```python
from build123d import *

# Parameters (mm, degrees)
SKETCH2_W             = 10
SKETCH2_H             = 14
SKETCH2_R             = 2.1
BOSS_EXTRUDE1_DEPTH   = 5
BOSS_EXTRUDE1_2_DEPTH = 5
SKETCH3_W             = 44.5
SKETCH3_H             = 39
SKETCH3_W_2           = 14
SKETCH3_H_2           = 5
BOSS_EXTRUDE2_DEPTH   = 2
BOSS_EXTRUDE4_DEPTH   = 32
SKETCH5_W             = 2
SKETCH5_H             = 85
BOSS_EXTRUDE5_DEPTH   = 37
SKETCH6_W             = 14
SKETCH6_H             = 30
CUT_EXTRUDE1_DEPTH    = 200
SKETCH7_W             = 20
SKETCH7_H             = 20
CUT_EXTRUDE2_DEPTH    = 16
FILLET1_R             = 2
SKETCH8_W             = 119.619460544
SKETCH8_H             = 55.607641494
CUT_EXTRUDE3_DEPTH    = 32
SKETCH9_W             = 100
SKETCH9_H             = 35
BOSS_EXTRUDE6_DEPTH   = 2
SKETCH10_W            = 89
SKETCH10_H            = 4
CUT_EXTRUDE4_DEPTH    = 10
BOSS_EXTRUDE7_DEPTH   = 25
SKETCH12_W            = 2
SKETCH12_H            = 35
BOSS_EXTRUDE8_DEPTH   = 2
SKETCH13_W            = 104
SKETCH13_H            = 37
BOSS_EXTRUDE9_DEPTH   = 2
SKETCH14_W            = 13
SKETCH14_H            = 30
CUT_EXTRUDE5_DEPTH    = 104
SKETCH15_W            = 13
SKETCH15_H            = 25
CUT_EXTRUDE7_DEPTH    = 120


with BuildPart() as part:
    # Sketch2 → Boss-Extrude1 (new body)
    with BuildSketch(Plane(origin=(0, 0, 0), x_dir=(1, 0, 0), z_dir=(0, 1, 0))):
        with Locations((114.448385229, -132.360414745)):
            Rectangle(SKETCH2_W, SKETCH2_H)
        with Locations((114.448385229, -132.360414745)):
            Circle(SKETCH2_R, mode=Mode.SUBTRACT)
    extrude(amount=BOSS_EXTRUDE1_DEPTH)



with BuildPart() as body_2:
    # Sketch2 → Boss-Extrude1 2 (new body)
    with BuildSketch(Plane(origin=(0, 0, 0), x_dir=(1, 0, 0), z_dir=(0, 1, 0))):
        with Locations((114.448385229, -172.360414745)):
            Rectangle(SKETCH2_W, SKETCH2_H)
        with Locations((114.448385229, -172.360414745)):
            Circle(SKETCH2_R, mode=Mode.SUBTRACT)
    extrude(amount=BOSS_EXTRUDE1_2_DEPTH)


with BuildPart() as part_1:
    add(part.part)

    add(body_2.part)  # Boss-Extrude2 merges body 2
    # Sketch3 → Boss-Extrude2 (add)
    with BuildSketch(Plane(origin=(119.448385229, 0, 0), x_dir=(0, 0, -1), z_dir=(1, 0, 0))):
        Polygon((-152.360414745, -34), (-152.360414745, 5), (-165.360414745, 5), (-165.360414745, 0), (-179.360414745, 0), (-179.360414745, 5), (-196.860414745, 5), (-196.860414745, -34), align=None)
        with Locations((-130.110414745, -14.5)):
            Rectangle(SKETCH3_W, SKETCH3_H)
        with Locations((-172.360414745, 2.5)):
            Rectangle(SKETCH3_W_2, SKETCH3_H_2)
    extrude(amount=BOSS_EXTRUDE2_DEPTH)

    # Sketch4 → Boss-Extrude4 (add)
    with BuildSketch(Plane(origin=(121.448385229, 0, 0), x_dir=(0, 0, -1), z_dir=(1, 0, 0))):
        Polygon((-194.860414745, 5), (-196.860414745, 5), (-196.860414745, -34), (-107.860414745, -34), (-107.860414745, 5), (-109.860414745, 5), (-109.860414745, -32), (-194.860414745, -32), align=None)
    extrude(amount=BOSS_EXTRUDE4_DEPTH)

    # Sketch5 → Boss-Extrude5 (add)
    with BuildSketch(Plane(origin=(0, -32, 0), x_dir=(1, 0, 0), z_dir=(0, 1, 0))):
        with Locations((152.448385229, -152.360414745)):
            Rectangle(SKETCH5_W, SKETCH5_H)
    extrude(amount=BOSS_EXTRUDE5_DEPTH)

    # Sketch6 → Cut-Extrude1 (cut)
    with BuildSketch(Plane.XY.offset(196.860414745)):
        with Locations((136.448385229, -10)):
            Rectangle(SKETCH6_W, SKETCH6_H)
    extrude(amount=-CUT_EXTRUDE1_DEPTH, mode=Mode.SUBTRACT)

    # Sketch7 → Cut-Extrude2 (cut)
    with BuildSketch(Plane(origin=(153.448385229, 0, 0), x_dir=(0, 0, -1), z_dir=(1, 0, 0))):
        with Locations((-179.360414745, -14.5)):
            Rectangle(SKETCH7_W, SKETCH7_H)
        with Locations((-152.360414745, -14.5)):
            Rectangle(SKETCH7_W, SKETCH7_H)
        with Locations((-125.360414745, -14.5)):
            Rectangle(SKETCH7_W, SKETCH7_H)
    extrude(amount=-CUT_EXTRUDE2_DEPTH, mode=Mode.SUBTRACT)

    # Fillet1
    fillet1_edges = [part_1.edges().sort_by_distance(p)[0] for p in [
        (109.448385229, 2.5, 139.360414745),
        (109.448385229, 2.5, 125.360414745),
        (109.448385229, 2.5, 179.360414745),
        (109.448385229, 2.5, 165.360414745),
    ]]
    fillet(fillet1_edges, radius=FILLET1_R)

    # Sketch8 → Cut-Extrude3 (cut)
    with BuildSketch(Plane(origin=(153.448385229, 0, 0), x_dir=(0, 0, -1), z_dir=(1, 0, 0))):
        with Locations((-148.578534845, -15.335015755)):
            Rectangle(SKETCH8_W, SKETCH8_H)
    extrude(amount=-CUT_EXTRUDE3_DEPTH, mode=Mode.SUBTRACT)

    # Sketch9 → Boss-Extrude6 (add)
    with BuildSketch(Plane(origin=(121.448385229, 0, 0), x_dir=(0, 0, -1), z_dir=(1, 0, 0))):
        with Locations((-152.360414745, -12.5)):
            Rectangle(SKETCH9_W, SKETCH9_H)
    extrude(amount=-BOSS_EXTRUDE6_DEPTH)

    # Sketch10 → Cut-Extrude4 (cut)
    with BuildSketch(Plane(origin=(121.448385229, 0, 0), x_dir=(0, 0, -1), z_dir=(1, 0, 0))):
        with Locations((-152.360414745, -32)):
            Rectangle(SKETCH10_W, SKETCH10_H)
    extrude(amount=-CUT_EXTRUDE4_DEPTH, mode=Mode.SUBTRACT)



with BuildPart() as body_2_2:
    # Sketch11 → Boss-Extrude7 (new body)
    with BuildSketch(Plane(origin=(121.448385229, 0, 0), x_dir=(0, 0, -1), z_dir=(1, 0, 0))):
        Polygon((-202.360414745, -30), (-202.360414745, 5), (-204.360414745, 5), (-204.360414745, -32), (-100.360414745, -32), (-100.360414745, 5), (-102.360414745, 5), (-102.360414745, -30), align=None)
    extrude(amount=BOSS_EXTRUDE7_DEPTH)


with BuildPart() as part_2:
    add(part_1.part)

    add(body_2_2.part)  # Boss-Extrude8 merges body 2 2
    # Sketch12 → Boss-Extrude8 (add)
    with BuildSketch(Plane.ZY.offset(-121.448385229)):
        with Locations((101.360414745, -12.5)):
            Rectangle(SKETCH12_W, SKETCH12_H)
        Polygon((102.360414745, -30), (100.360414745, -30), (100.360414745, -32), (204.360414745, -32), (204.360414745, -30), (202.360414745, -30), align=None)
        with Locations((203.360414745, -12.5)):
            Rectangle(SKETCH12_W, SKETCH12_H)
    extrude(amount=BOSS_EXTRUDE8_DEPTH)

    # Sketch13 → Boss-Extrude9 (add)
    with BuildSketch(Plane(origin=(146.448385229, 0, 0), x_dir=(0, 0, -1), z_dir=(1, 0, 0))):
        with Locations((-152.360414745, -13.5)):
            Rectangle(SKETCH13_W, SKETCH13_H)
        Polygon((-195.798080738, -22), (-175.798080738, -22), (-185.798080738, -0.554930795), align=None, mode=Mode.SUBTRACT)
        Polygon((-128.922748753, -22), (-118.922748753, -0.554930795), (-108.922748753, -22), align=None, mode=Mode.SUBTRACT)
        Polygon((-162.360414745, -22), (-142.360414745, -22), (-152.360414745, -0.554930795), align=None, mode=Mode.SUBTRACT)
    extrude(amount=BOSS_EXTRUDE9_DEPTH)

    # Sketch14 → Cut-Extrude5 (cut)
    with BuildSketch(Plane(origin=(0, 0, 100.360414745), x_dir=(-1, 0, 0), z_dir=(0, 0, -1))):
        with Locations((-133.948385229, 5)):
            Rectangle(SKETCH14_W, SKETCH14_H)
    extrude(amount=-CUT_EXTRUDE5_DEPTH, mode=Mode.SUBTRACT)

    # Sketch15 → Cut-Extrude7 (cut)
    with BuildSketch(Plane(origin=(0, 0, 100.360414745), x_dir=(-1, 0, 0), z_dir=(0, 0, -1))):
        with Locations((-133.948385229, -7.5)):
            Rectangle(SKETCH15_W, SKETCH15_H)
    extrude(amount=-CUT_EXTRUDE7_DEPTH, mode=Mode.SUBTRACT)


solid = part_2.part
```
For this review, take the finished solid that the model builds, in its own axes (mm). A direction names the side the tool comes from. Give positions to 0.01 mm unless a question says otherwise; leave off trailing zeros. Order: outer loops, then holes, each group sorted by start corner. A loop starts at its lowest first (then second) coordinate and runs counter-clockwise, first axis right, second up.
1) Take a section at A-A (x = 118.5). Give the boundary of the cut face in (y, z).
2) Insertion check: pin 1 (5 mm diameter, centred on y = -26.5, z = 121, fed in from -X); pin 2 (1.6 mm diameter, centred on x = 133.5, z = 101.5, fed in from +Y); pin 3 (5.5 mm diameter, centred on x = 115, y = 1.5, fed in from -Z). Each pin has a flat end and moves straight along its axis. Give the tip position at first contact, or say it passes through.
3) For faces 1 (the face through (127.448, -8, 101)), 2 (the face through (110.05, 2.54, 138.79)), 3 (the face through (134, -21, 202.36)), 4 (the face through (147.43, -11.13, 157.29)), list the 3-axis set-ups (+Z, -Z, +X, -X, +Y, -Y) from which the entire face can be reached by the end or side of a thin tool; tool diameter is ignored.
4) The part is to be moulded in two halves that separate along Z. For faces 5 (the face through (115.58, 2.46, 130.59)), 6 (the face through (147.43, -11.13, 190.73)), 7 (the face through (109.448, 2, 172)), 8 (the face through (110.02, 2.54, 125.96)), say which applies: released by +Z, released by -Z, zero draft, split by the parting line, or undercut.
5) Wall thickness on line 1 (Z direction, x = 127, y = -9.5); line 2 (X direction, y = -6.5, z = 141.5); line 3 (Z direction, x = 112, y = 4): over which ranges is each line inside the solid? List them lowest first.
6) Take a section at D-D (z = 149.5). Give the boundary of the cut face in (x, y), then the cut area to 3 significant figures.
7) Take a section at B-B (y = -23). Give the boundary of the cut face in (x, z), then the cut area to 3 significant figures.
8) Take a section at C-C (y = 2.5). State how many separate pieces and enclosed holes the cut face has, then the cut area to 3 significant figures.
Derived:
1. outline: (0, 125.36) - (5, 125.36) - (5, 139.36) - (0, 139.36) - close; (0, 165.36) - (5, 165.36) - (5, 179.36) - (0, 179.36) - close
2. pin 1: stops at x = 119.45
2. pin 2: stops at y = -20
2. pin 3: stops at z = 125.36
3. face 1: +Z, -Z, +Y
3. face 2: -X, +Y, -Y
3. face 3: +Y
3. face 4: +X
4. face 5: undercut
4. face 6: undercut
4. face 7: zero draft
4. face 8: released by -Z
5. line 1: z = 100.36 to 102.36, 202.36 to 204.36
5. line 2: x = 119.45 to 121.45, 146.45 to 148.45
5. line 3: z = 125.36 to 139.36, 165.36 to 179.36
6. outline: (119.45, -32) - (148.45, -32) - (148.45, -22) - (146.45, -22) - (146.45, -30) - (121.45, -30) - (121.45, 5) - (119.45, 5) - close; (146.45, -6.69) - (148.45, -6.69) - (148.45, 5) - (146.45, 5) - close
6. area: 167 mm2
7. outline: (119.45, 100.36) - (148.45, 100.36) - (148.45, 204.36) - (119.45, 204.36) - close; hole (121.45, 102.36) - (146.45, 102.36) - (146.45, 202.36) - (121.45, 202.36) - close
7. area: 516 mm2
8. separate pieces: 2
8. enclosed holes: 2
8. area: 713 mm2
